from build123d import *

# Parameters (mm, degrees)
SKETCH_W      = 30
SKETCH_H      = 12
PAD_DEPTH     = 20
PAD001_DEPTH  = 5
SKETCH002_R   = 1.5
PAD002_DEPTH  = 5
CHAMFER_SIZE2 = 15
CHAMFER_SIZE  = 10
FILLET_R      = 2


with BuildPart() as part:
    # Sketch → Pad (new body)
    with BuildSketch(Plane.XY):
        with Locations((15, 6)):
            Rectangle(SKETCH_W, SKETCH_H)
    extrude(amount=PAD_DEPTH)

    # Sketch001 (on Face5 of Pad) → Pad001 (join)
    with BuildSketch(Plane(origin=(0, 0, 0), x_dir=(1, 0, 0), z_dir=(0, 0, -1))):
        Polygon((12, 0), (18, 0), (18, -3), (20, -3), (20, -8), (10, -8), (10, -3), (12, -3), align=None)
    extrude(amount=PAD001_DEPTH)

    # Sketch002 (on Face4 of Pad001) → Pad002 (join)
    with BuildSketch(Plane(origin=(0, 0, 0), x_dir=(1, 0, 0), z_dir=(0, 0, -1))):
        with Locations((3.5, -6)):
            Circle(SKETCH002_R)
        with Locations((26.5, -6)):
            Circle(SKETCH002_R)
    extrude(amount=PAD002_DEPTH)

    # Chamfer
    chamfer_edges = [part.edges().sort_by_distance(p)[0] for p in [
        (15, 12, 20),
    ]]
    chamfer_side = part.faces().sort_by_distance((15, 6, 20))[0]
    chamfer(chamfer_edges, length=CHAMFER_SIZE, length2=CHAMFER_SIZE2, reference=chamfer_side)

    # Fillet
    fillet_edges = [part.edges().sort_by_distance(p)[0] for p in [
        (0, 12, 2.5),
        (0, 0, 10),
        (30, 12, 2.5),
        (30, 0, 10),
    ]]
    fillet(fillet_edges, radius=FILLET_R)


solid = part.part
Geometry check sheet. Reference: the model listing, model coordinates, mm. A direction names the side the tool comes from. Round coordinates to 2 decimals unless told otherwise and drop trailing zeros. Loops run counter-clockwise (first coordinate to the right, second up) from the corner with the lowest first, then second, coordinate; pieces in that order, holes last. Notation, with made-up numbers: (-32, 85) -> (3, 85) arc R22 cw to (3, 113) -> close; hole circle Ø5 at (62, 39). An arc over 180 degrees is marked (long way). Answer as a JSON object with one key per item and string values. Group by question number.
Item 1: Set-up check for faces 1 (the face through (3, 6, -5)), 2 (the face through (11, 3, -2)), 3 (the face through (18, 1, -2)): record each of +Z, -Z, +X, -X, +Y, -Y from which the full face is reachable in a straight line by a thin tool's end or side.
Item 2: Thickness scan on line 1 along Y through (x, z) = (7, 18.5); line 2 along Z through (x, y) = (16.25, 7.5); line 3 along Z through (x, y) = (3.25, 10). Record the ranges inside material, lowest first.
Item 3: Cross-section at A-A, the plane z = 11.75. Record the cut outline in (x, y), plus the area to 3 significant figures.
Item 4: Cross-section at D-D, the plane x = 26.5. Record the cut outline in (y, z), plus the area to 3 significant figures.
Item 5: Cross-section at C-C, the plane x = 15.75. Record the cut outline in (y, z), plus the area to 3 significant figures.
Item 6: Cross-section at B-B, the plane y = 3.5. Record the cut outline in (x, z).
Item 7: Release check for a two-part mould opening along X. For faces 4 (the face through (15, 8, -2)), 5 (the face through (10, 6, -2)), 6 (the face through (30, 5, 8)) record: pulls with the +X half, pulls with the -X half, needs draft (parallel to the pull), parting line crosses it, or undercut.
Item 8: Depth check by flat-ended pin: pin 1 Ø2.5 at (y, z) = (2, -2.5) entering from -X; pin 2 Ø3 at (x, y) = (24.5, 8.5) entering from -Z; pin 3 Ø4 at (x, z) = (17, 8.5) entering from +Y; pin 4 Ø1.5 at (x, z) = (17, -0.5) entering from -Y. Enter the tip coordinate at first touch or a pass-through.
Determined:
{
 "1": {"face 1": "-Z, +X, -X, +Y, -Y", "face 2": "-Z, -X, -Y", "face 3": "-Z, +X, -Y"},
 "2": {"line 1": "y = 0 to 3", "line 2": "z = -5 to 11.75", "line 3": "z = 0 to 8"},
 "3": {"outline": "(0, 2) arc R2 ccw to (2, 0) -> (28, 0) arc R2 ccw to (30, 2) -> (30, 7.5) -> (0, 7.5) -> close", "area": "223 mm²"},
 "4": {"outline": "(0, 0) -> (4.5, 0) -> (4.5, -5) -> (7.5, -5) -> (7.5, 0) -> (12, 0) -> (12, 5) -> (2, 20) -> (0, 20) -> close", "area": "180 mm²"},
 "5": {"outline": "(0, -5) -> (8, -5) -> (8, 0) -> (12, 0) -> (12, 5) -> (2, 20) -> (0, 20) -> close", "area": "205 mm²"},
 "6": {"outline": "(0, 0) -> (10, 0) -> (10, -5) -> (20, -5) -> (20, 0) -> (30, 0) -> (30, 17.75) -> (0, 17.75) -> close"},
 "7": {"face 4": "needs draft", "face 5": "undercut", "face 6": "pulls with the +X half"},
 "8": {"pin 1": "stops at x = 10", "pin 2": "stops at z = 0", "pin 3": "stops at y = 11", "pin 4": "stops at y = 0"}
}
